Autodesk Inventor part; units mm, degrees
ref_plane "YZ Plane" through (0, 0, 0) normal (1, 0, 0) x (0, 1, 0)
ref_plane "XZ Plane" through (0, 0, 0) normal (0, 1, 0) x (-1, 0, 0)
ref_plane "XY Plane" through (0, 0, 0) normal (0, 0, 1) x (1, 0, 0)
sketch "スケッチ1" plane through (0, 0, 0) normal (0, 0, 1) x (1, 0, 0)
  circle A0 centre (0, 0) radius 3
  dimension "d0" = 6
extrude "押し出し1" add sketch "スケッチ1" along normal blind 35
hole "穴1" at (0, 0, 0) direction (0, 0, 1) diameter 3 depth 6 tip angle 118
sketch "スケッチ2" plane through (0, 0, 35) normal (0, 0, 1) x (1, 0, 0)
  circle A0 centre (0, 0) radius 3
hole "穴2" at (0, 0, 35) direction (0, 0, -1) diameter 3 depth 6 tip angle 118
properties part number "スペーサ　l35" material "アルミニウム 2014-T4"
Part model, mm, in its own coordinate system. A direction names the side the tool comes from. Round coordinates to 2 decimals unless told otherwise and drop trailing zeros. Order: outer loops, then holes, each group sorted by start corner. A loop starts at its lowest first (then second) coordinate and runs counter-clockwise, first axis right, second up. Notation, with made-up numbers: M 55,-25.5 L 111,-25.5 A33 cw 111,4.5 Z; hole C 84.5,-36 d3. An arc over 180 degrees is marked long. Answer in a Markdown table with one row per item. Add a question column.
Q1. Mould opens along X. For faces 1 (the face through (-3, 0, 17)), 2 (the face through (1.3, -1.3, 35)), 3 (the face through (-0.07, 1.5, 31.96)) say: +X half, -X half, draft (parallel to the pull), parting line (faces both ways), or undercut.
Q2. Cut at A-A on z = 12. Give the cut face in (x, y).
Q3. Pin check, flat tips, straight feed: pin 1 (1.8 mm diameter, centred on x = 0, y = 0, fed in from +Z); pin 2 (1 mm diameter, centred on x = 2, z = 11, fed in from -Y); pin 3 (2.5 mm diameter, centred on x = 0, y = 0, fed in from -Z). Stop position of each tip, or through.
Q4. 3-axis set-ups, long thin cutter, end or side, ignore diameter. For faces 4 (the face through (-0.07, -1.5, 3.04)), 5 (the face through (1.3, -1.3, 0)): which of +Z, -Z, +X, -X, +Y, -Y reach the whole face in a straight line?
Q5. Wall check: L1, parallel to Y at x = 0, z = 32.7; L2, parallel to X at y = -1.2, z = 33.5; L3, parallel to Y at x = 2.65, z = 32.5. Give the ranges that are in metal, low to high. Write a range as from..to.
Established:
| question | item | result |
|---|---|---|
| 1 | face 1 | parting line |
| 1 | face 2 | draft |
| 1 | face 3 | undercut |
| 2 | outline | C 0,0 d6 |
| 3 | pin 1 | stops at z = 28.64 |
| 3 | pin 2 | stops at y = -2.6 |
| 3 | pin 3 | stops at z = 6.15 |
| 4 | face 4 | -Z |
| 4 | face 5 | -Z, +X, -X, +Y, -Y |
| 5 | L1 | y = -3..-1.5, 1.5..3 |
| 5 | L2 | x = -2.75..-0.9, 0.9..2.75 |
| 5 | L3 | y = -1.41..1.41 |
